Input: dimensioned drawing with shaded views. Units: mm. Origin: part minimum x, y, z. A direction names the side the tool comes from. Coordinates: 2 decimals unless noted, no trailing zeros. Order: outer loops, then holes, each group sorted by start corner. A loop starts at its lowest first (then second) coordinate and runs counter-clockwise, first axis right, second up. Notation, with made-up numbers: (67.25, -15.75) - (94.25, -15.75) arc R33 ccw to (94.25, 20.25) - close; hole circle Ø11 at (55, 52). An arc over 180 degrees is marked (long way). One line per question, with ' | ' between items. Start each with the question number.
(1) Line query: line 1 along Z through (x, y) = (14.5, 12.5); line 2 along Y through (x, z) = (10, 2); line 3 along X through (y, z) = (11.25, 23.25). Output: solid intervals per line, ascending.
(2) Contact query for flat-ended pins moving along their axis: P1, Ø5, axis at x = 15, y = 5.5, coming from the +Z side; P2, Ø2, axis at x = 17, z = 13, coming from the -Y side; P3, Ø1.5, axis at x = 8, z = 4.5, coming from the +Y side; P4, Ø1, axis at y = 8, z = 3, coming from the -X side. Output: stop coordinate, or through.
(3) Access query for the marked faces 1, 2 and 3. Directions: +Z, -Z, +X, -X, +Y, -Y. A direction counts if a zero-diameter tool reaches every point of the face in a straight line with its end or side. Return the directions, or none.
(4) Section A-A (x = 10). Return the cut outline in (y, z), then the cut area to 3 significant figures.
(5) Section D-D (y = 2). Return the cut outline in (x, z).
(6) Section C-C (z = 10). Return the cut outline in (x, y), then the cut area to 3 significant figures.
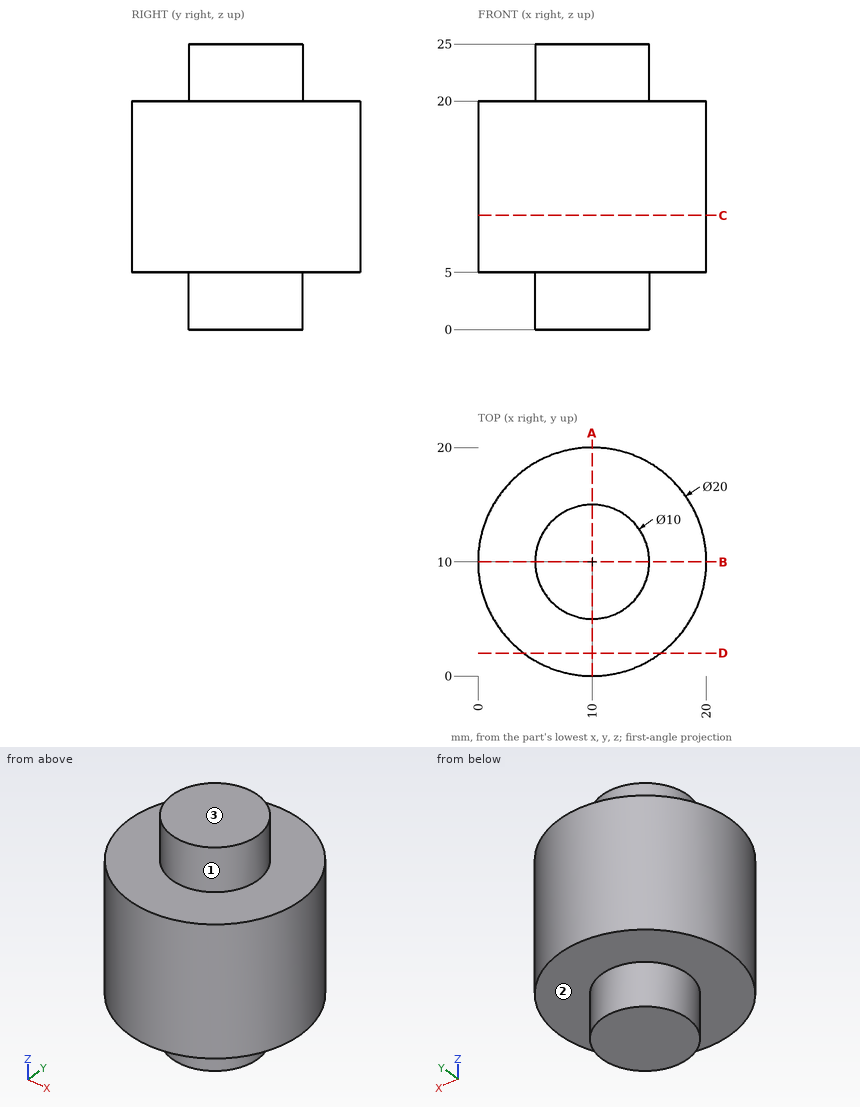
Response values:
1) line 1: z = 5 to 20 | line 2: y = 5 to 15 | line 3: x = 5.16 to 14.84
2) P1: stops at z = 25 | P2: stops at y = 2 | P3: stops at y = 19.9 | P4: stops at x = 5.23
3) face 1: +Z | face 2: -Z | face 3: +Z, +X, -X, +Y, -Y
4) outline: (0, 5) - (5, 5) - (5, 0) - (15, 0) - (15, 5) - (20, 5) - (20, 20) - (15, 20) - (15, 25) - (5, 25) - (5, 20) - (0, 20) - close | area: 400 mm²
5) outline: (4, 5) - (16, 5) - (16, 20) - (4, 20) - close
6) outline: circle Ø20 at (10, 10) | area: 314 mm²
